For this review, use the dimensioned drawing (mm, ordinates from the lowest corner) and the shaded views. Round coordinates to 2 decimals unless told otherwise and drop trailing zeros. Write each loop counter-clockwise with the first axis right and the second up, starting at its lowest first coordinate (ties: lowest second). Pieces come first, ordered by that corner, then holes. Notation, with made-up numbers: M 56.25,62.5 L 87.25,62.5 A22 cw 87.25,79.5 Z; hole C 78,59.5 d5. An arc over 180 degrees is marked long. One line per question, with ' | ' between items.
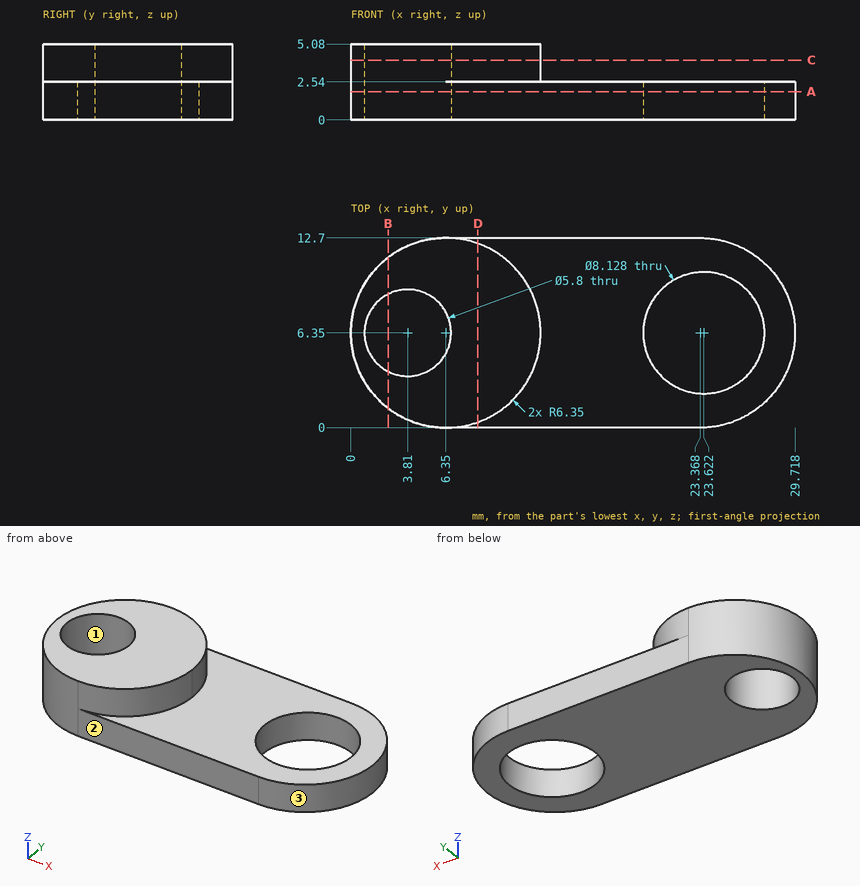
Item 1: Take a section at D-D (x = 8.5). Write out the cut boundary in (y, z).
Results:
outline: M 0,0 L 12.7,0 L 12.7,2.54 L 12.32,2.54 L 12.32,5.08 L 0.38,5.08 L 0.38,2.54 L 0,2.54 Z
Item 2: Mouldability with a two-part tool opening along X and no side actions: class the marked faces 1, 2 and 3 as +X half, -X half, draft (parallel to the pull), parting line (faces both ways), or undercut.
Results:
face 1: undercut | face 2: draft | face 3: +X half
Item 3: Take a section at B-B (x = 2.5). Write out the cut boundary in (y, z), then the cut area to 3 significant figures.
Results:
outline: M 1.3,0 L 3.76,0 L 3.76,5.08 L 1.3,5.08 Z; M 8.94,0 L 11.4,0 L 11.4,5.08 L 8.94,5.08 Z | area: 25.0 mm2
Item 4: Insertion check: pin 1 Ø1.5 at (y, z) = (5, 4) entering from +X; pin 2 Ø3.5 at (x, y) = (3.81, 6.35) entering from +Z; pin 3 Ø1 at (y, z) = (7.5, 2.5) entering from -X; pin 4 Ø4 at (x, y) = (21, 5) entering from +Z. Each pin has a flat end and moves straight along its axis. Give the tip position at first contact, or say it passes through.
Results:
pin 1: x = 12.67 | pin 2: through | pin 3: x = 0.03 | pin 4: z = 2.54
Item 5: Take a section at C-C (z = 4). Write out the cut boundary in (x, y), then the cut area to 3 significant figures.
Results:
outline: C 6.35,6.35 d12.7; hole C 3.81,6.35 d5.8 | area: 100 mm2
Item 6: Take a section at A-A (z = 1.9). Write out the cut boundary in (x, y), then the cut area to 3 significant figures.
Results:
outline: M 6.35,0 L 23.37,0 A6.35 ccw 23.37,12.7 L 6.35,12.7 A6.35 ccw Z; hole C 3.81,6.35 d5.8; hole C 23.62,6.35 d8.13 | area: 264 mm2
Item 7: To check wall thickness, follow line 1 along X through (y, z) = (4.25, 0.4); line 2 along Z through (x, y) = (14.75, 7); line 3 along Y through (x, z) = (3.81, 1.75). State the ranges of each line that lie inside material, in increasing order. Write a range as from..to.
Results:
line 1: 0.36..1.81, 5.81..20.14, 27.1..29.36 | line 2: 0..2.54 | line 3: 0.53..3.45, 9.25..12.17
